Part model, mm, in its own coordinate system. A direction names the side the tool comes from. Coordinates: 2 decimals unless noted, no trailing zeros. Loops run counter-clockwise (first coordinate to the right, second up) from the corner with the lowest first, then second, coordinate; pieces in that order, holes last. Notation, with made-up numbers: M -12.75,8 L 8.25,8 A18 ccw 8.25,41 Z; hole C 57.25,-24 d5. An arc over 180 degrees is marked long. Answer as a JSON object with one key per item and string values. Group by question number.
1. Saw through at D-D on x = 4.5. Write the cut outline in (y, z) (3 decimals), then the cut area to 3 significant figures.
2. Saw through at B-B on y = 7.25. Write the cut outline in (x, z) (3 decimals).
3. 3-axis set-ups, long thin cutter, end or side, ignore diameter. For faces 5 (the face through (26.67, 1, 0)), 6 (the face through (7.62, 1, 15)), 7 (the face through (-13.97, 2, -14)): which of +Z, -Z, +X, -X, +Y, -Y reach the whole face in a straight line?
4. Saw through at C-C on z = 9.5. Write the cut outline in (x, y).
5. Drill centre lines: L1, parallel to X at y = 6, z = -7.5; L2, parallel to Y at x = -19.05, z = -5; L3, parallel to X at y = 8, z = 4.5. Where is each one in solid material? Low to high.
6. Saw through at A-A on x = -21.5. Write the cut outline in (y, z) (3 decimals).
7. Drop flat-ended pins along their axis: pin 1 Ø0.8 at (y, z) = (0.5, 14.5) entering from -X; pin 2 Ø9.5 at (x, z) = (12, 3) entering from +Y; pin 3 Ø0.8 at (x, y) = (-28, 2) entering from -Z; pin 4 Ø3 at (x, y) = (13.5, 10) entering from -Z. Give the stop position or say it passes through.
8. Mould opens along Z. For faces 1 (the face through (-10.16, 1, 15)), 2 (the face through (0, 1, 15.875)), 3 (the face through (28, 1, -1.27)), 4 (the face through (-26.67, 1, 0)) say: released by +Z, released by -Z, zero draft, split by the parting line, or undercut.
from build123d import *

# Parameters (mm, degrees)
SKETCH1_W           = 58.42
SKETCH1_H           = 31.75
BOSS_EXTRUDE1_DEPTH = 2.54
FILLET1_R           = 2.54
SKETCH4_R           = 5.08
BOSS_EXTRUDE3_DEPTH = 15.875
SKETCH5_R           = 5.08
BOSS_EXTRUDE4_DEPTH = 10.16
SKETCH6_R           = 3.556
CUT_EXTRUDE2_DEPTH  = 32.75
SKETCH9_W           = 13.97
SKETCH9_H           = 3.81
CUT_EXTRUDE4_DEPTH  = 1.27
SKETCH10_W          = 2.54
SKETCH10_H          = 2.54
SKETCH10_W_2        = 20.32
SKETCH10_H_2        = 3.81
CUT_EXTRUDE6_DEPTH  = 12.176


with BuildPart() as part:
    # Sketch1 → Boss-Extrude1 (new body)
    with BuildSketch(Plane(origin=(0, 0, 0), x_dir=(1, 0, 0), z_dir=(0, 1, 0))):
        Rectangle(SKETCH1_W, SKETCH1_H)
    extrude(amount=BOSS_EXTRUDE1_DEPTH)

    # Fillet1
    fillet1_edges = [part.edges().sort_by_distance(p)[0] for p in [
        (29.21, 1.27, 15.875),
        (-29.21, 1.27, 15.875),
        (-29.21, 1.27, -15.875),
        (29.21, 1.27, -15.875),
    ]]
    fillet(fillet1_edges, radius=FILLET1_R)

    # Sketch4 → Boss-Extrude3 (add)
    with BuildSketch(Plane.XY):
        with Locations((-19.05, 6.096)):
            Circle(SKETCH4_R)
        with Locations((19.05, 6.096)):
            Circle(SKETCH4_R)
    extrude(amount=BOSS_EXTRUDE3_DEPTH)

    # Sketch5 → Boss-Extrude4 (add)
    with BuildSketch(Plane(origin=(0, 0, 0), x_dir=(-1, 0, 0), z_dir=(0, 0, -1))):
        with Locations((-19.05, 6.096)):
            Circle(SKETCH5_R)
        with Locations((19.05, 6.096)):
            Circle(SKETCH5_R)
    extrude(amount=BOSS_EXTRUDE4_DEPTH)

    # Sketch6 → Cut-Extrude2 (cut, through all)
    with BuildSketch(Plane.XY.offset(15.875)):
        with Locations((-19.05, 6.096)):
            Circle(SKETCH6_R)
        with Locations((19.05, 6.096)):
            Circle(SKETCH6_R)
    extrude(amount=-CUT_EXTRUDE2_DEPTH, mode=Mode.SUBTRACT)

    # Sketch9 → Cut-Extrude4 (cut)
    with BuildSketch(Plane(origin=(0, 2.54, 0), x_dir=(1, 0, 0), z_dir=(0, 1, 0))):
        with Locations((-6.985, 13.97)):
            Rectangle(SKETCH9_W, SKETCH9_H)
        with Locations((6.985, 13.97)):
            Rectangle(SKETCH9_W, SKETCH9_H)
    extrude(amount=-CUT_EXTRUDE4_DEPTH, mode=Mode.SUBTRACT)

    # Sketch10 → Cut-Extrude6 (cut, through all)
    with BuildSketch(Plane(origin=(0, 0, 0), x_dir=(1, 0, 0), z_dir=(0, 1, 0))):
        with Locations((-27.94, 0)):
            Rectangle(SKETCH10_W, SKETCH10_H)
        with Locations((27.94, 0)):
            Rectangle(SKETCH10_W, SKETCH10_H)
        with Locations((0, 13.97)):
            Rectangle(SKETCH10_W_2, SKETCH10_H_2)
        with Locations((-8.89, -14.605)):
            Rectangle(SKETCH10_W, SKETCH10_H)
        with Locations((8.89, -14.605)):
            Rectangle(SKETCH10_W, SKETCH10_H)
    extrude(amount=CUT_EXTRUDE6_DEPTH, mode=Mode.SUBTRACT)


solid = part.part
Outcome:
{
 "1": {"outline": "M 0,-12.065 L 2.54,-12.065 L 2.54,15.875 L 0,15.875 Z", "area": "71.0 mm²"},
 "2": {"outline": "M -23.997,-10.16 L -22.414,-10.16 L -22.414,15.875 L -23.997,15.875 Z; M -15.686,-10.16 L -14.103,-10.16 L -14.103,15.875 L -15.686,15.875 Z; M 14.103,-10.16 L 15.686,-10.16 L 15.686,15.875 L 14.103,15.875 Z; M 22.414,-10.16 L 23.997,-10.16 L 23.997,15.875 L 22.414,15.875 Z"},
 "3": {"face 5": "+X, +Y, -Y", "face 6": "+Z, +Y, -Y", "face 7": "-Z, +Y"},
 "4": {"outline": "M -29.21,0 L 29.21,0 L 29.21,2.54 L 22.68,2.54 A5.08 ccw long 15.42,2.54 L -15.42,2.54 A5.08 ccw long -22.68,2.54 L -29.21,2.54 Z; hole C -19.05,6.1 d7.11; hole C 19.05,6.1 d7.11"},
 "5": {"L1": "x = -24.13 to -22.6, -15.5 to -13.97, 13.97 to 15.5, 22.6 to 24.13", "L2": "y = 0 to 2.54, 9.65 to 11.18", "L3": "x = -23.76 to -22.05, -16.05 to -14.34, 14.34 to 16.05, 22.05 to 23.76"},
 "6": {"outline": "M 0,-15.875 L 2.54,-15.875 L 2.54,-10.16 L 3.519,-10.16 L 3.519,15.875 L 0,15.875 Z; M 8.673,-10.16 L 10.546,-10.16 L 10.546,15.875 L 8.673,15.875 Z"},
 "7": {"pin 1": "stops at x = -29.09", "pin 2": "stops at y = 10.63", "pin 3": "stops at z = -15.7", "pin 4": "passes through"},
 "8": {"face 1": "zero draft", "face 2": "released by +Z", "face 3": "undercut", "face 4": "undercut"}
}
